Geometry check sheet. Reference: the model listing, model coordinates, mm. A direction names the side the tool comes from. Coordinates: 2 decimals unless noted, no trailing zeros. Loops run counter-clockwise (first coordinate to the right, second up) from the corner with the lowest first, then second, coordinate; pieces in that order, holes last. Notation, with made-up numbers: (9, 23) - (44, 23) arc R19 cw to (44, 39) - close; hole circle Ø1 at (-4.75, 42). An arc over 180 degrees is marked (long way). One line per item, written item: value.
Autodesk Inventor part; units mm, degrees
ref_plane "YZ Plane" through (0, 0, 0) normal (1, 0, 0) x (0, 1, 0)
ref_plane "XZ Plane" through (0, 0, 0) normal (0, 1, 0) x (-1, 0, 0)
ref_plane "XY Plane" through (0, 0, 0) normal (0, 0, 1) x (1, 0, 0)
sketch "Sketch1" plane through (0, 0, 0) normal (0, 1, 0) x (-1, 0, 0)
  line L0 (0, 0) -> (15, 0)
  line L1 (15, 0) -> (15, -32)
  line L2 (15, -32) -> (0, -32)
  line L3 (0, -32) -> (0, 0)
  line L4 (3, 0) -> (12, 0)
  line L5 (12, 0) -> (12, 8)
  line L6 (12, 8) -> (3, 8)
  line L7 (3, 8) -> (3, 0)
  line L8 (-5, -32) -> (-5, 5)
  line L9 (-5, 5) -> (-2, 5)
  line L10 (-2, 5) -> (-2, 13)
  line L11 (-2, 13) -> (17, 13)
  line L12 (17, 13) -> (17, 5)
  line L13 (17, 5) -> (20, 5)
  line L14 (20, 5) -> (20, -37)
  line L15 (20, -37) -> (-5, -37)
  line L16 (-5, -37) -> (-5, -32)
  line L17 (-5, -8.634) -> (-25, -8.634)
  line L18 (-25, -8.634) -> (-25, -18.634)
  line L19 (-25, -18.634) -> (-5, -18.634)
  line L20 (-5, -18.634) -> (-5, -8.634)
  line L21 (20, -18.634) -> (40, -18.634)
  line L22 (40, -18.634) -> (40, -8.634)
  line L23 (40, -8.634) -> (20, -8.634)
  line L24 (20, -8.634) -> (20, -18.634)
  dimension "d0" = 15
  dimension "d1" = 32
  dimension "d2" = 9
  dimension "d3" = 3
  dimension "d4" = 3
  dimension "d5" = 8
  dimension "d6" = 5
  dimension "d7" = 5
  dimension "d8" = 5
  dimension "d9" = 5
  dimension "d10" = 5
  dimension "d11" = 5
  dimension "d12" = 5
  dimension "d13" = 5
  dimension "d71" = 20
  dimension "d72" = 10
  dimension "d73" = 20
  dimension "d74" = 10
extrude "Extrusion1" add sketch "Sketch1" along normal blind 10
sketch "Sketch3" plane through (5, 0, -37) normal (0, 0, -1) x (-1, 0, 0)
  line L0 (0.5, 10) -> (24.5, 10)
  line L1 (24.5, 10) -> (24.5, 1)
  line L2 (24.5, 1) -> (0.5, 1)
  line L3 (0.5, 1) -> (0.5, 10)
  line L4 (25, 0) -> (25, 10)
  line L5 (0, 0) -> (0, 10)
  line L6 (0, 0) -> (25, 0)
  line L7 (0, 10) -> (25, 10)
  point P0 (5, 0)
  point P1 (24.5, 5.5)
  dimension "d24" = 0.5
  dimension "d25" = 0.5
  dimension "d26" = 1
  dimension "d27" = 0
extrude "Extrusion3" cut sketch "Sketch3" against normal blind 10 contours L0 L1 L2 L3
sketch "Sketch4" plane through (-17, 0, 13) normal (0, 0, 1) x (1, 0, 0)
  line L0 (5, 10) -> (14, 10)
  line L1 (14, 10) -> (14, 2)
  line L2 (14, 2) -> (5, 2)
  line L3 (5, 2) -> (5, 10)
  line L4 (0, 0) -> (19, 0)
  line L5 (0, 10) -> (19, 10)
  line L6 (19, 0) -> (19, 10)
  line L7 (0, 0) -> (0, 10)
  point P0 (17, 0)
  point P1 (9.5, 0)
  dimension "d30" = 2
  dimension "d31" = 0
  dimension "d32" = 5
  dimension "d33" = 5
extrude "Extrusion4" cut sketch "Sketch4" against normal blind 10 contours L0 L1 L2 L3
sketch "Sketch5" plane through (0, 0, 0) normal (0, -1, 0) x (1, 0, 0)
  line L0 (-17, 5) -> (-17, 13)
  line L1 (2, 13) -> (2, 5)
  line L2 (-17, 13) -> (2, 13)
  line L3 (2, 13) -> (2, 5)
  line L4 (5, 5) -> (5, -37)
  line L5 (2, 5) -> (5, 5)
  line L6 (5, 5) -> (5, -37)
  line L7 (-20, -37) -> (-20, 5)
  line L8 (5, -37) -> (-20, -37)
  line L9 (-20, -37) -> (-20, 5)
  line L10 (-20, 5) -> (-17, 5)
  point P0 (0, 0)
extrude "Extrusion5" add sketch "Sketch5" along normal blind 5
sketch "Sketch6" plane through (0, 10, 0) normal (0, 1, 0) x (1, 0, 0)
  circle A0 centre (-18.5, 2.5) radius 1
  line L0 (-20, -5) -> (-17, -5)
  line L1 (-20, 37) -> (-20, -5)
  circle A1 centre (3.5, 2.5) radius 1
  line L2 (2, -5) -> (5, -5)
  line L3 (2, -13) -> (2, -5)
  point P0 (0, 0)
  dimension "d59" = 2
  dimension "d60" = 7.5
  dimension "d61" = 1.5
  dimension "d62" = 2
  dimension "d63" = 7.5
  dimension "d64" = 1.5
extrude "Extrusion6" cut sketch "Sketch6" against normal blind 5
thread "Thread1"
thread "Thread2"
sketch "Sketch7" plane through (25, 0, -18.634) normal (0, 0, -1) x (-1, 0, 0)
  point P0 (25, 0)
sketch "Sketch8" plane through (25, 0, -18.634) normal (0, 0, -1) x (-1, 0, 0)
  circle A0 centre (10, 5) radius 2
  circle A1 centre (55, 5) radius 2
  line L0 (65, 0) -> (65, 10)
  line L1 (0, 0) -> (0, 10)
  line L2 (0, 10) -> (20, 10)
  line L3 (45, 10) -> (65, 10)
  point P0 (25, 0)
  point P1 (65, 5)
  dimension "d76" = 4
  dimension "d77" = 4
  dimension "d78" = 10
  dimension "d79" = 10
  dimension "d80" = 5
  dimension "d81" = 5
extrude "Extrusion7" cut sketch "Sketch8" against normal blind 10
thread "Thread3"
thread "Thread4"
properties part number "Base"
(1) Release check for a two-part mould opening along Z. For faces 1 (the face through (-8, 1, 8)), 2 (the face through (-17, 6, -27)), 3 (the face through (15, 0, -14)) record: pulls with the +Z half, pulls with the -Z half, needs draft (parallel to the pull), parting line crosses it, or undercut.
Reply:
face 1: undercut
face 2: pulls with the -Z half
face 3: needs draft
(2) Cross-section at D-D on x = 3.5. Record the cut outline in (y, z).
Reply:
outline: (-5, -37) - (1, -37) - (1, -27) - (10, -27) - (10, -3.5) - (5, -3.5) - (5, -1.5) - (10, -1.5) - (10, 5) - (-5, 5) - close
(3) Cross-section at C-C on z = -13. Record the cut outline in (x, y), and give its area (3 significant figures).
Reply:
outline: (-40, 0) - (-20, 0) - (-20, -5) - (5, -5) - (5, 0) - (25, 0) - (25, 10) - (0, 10) - (0, 0) - (-15, 0) - (-15, 10) - (-40, 10) - close; hole circle Ø4 at (-30, 5); hole circle Ø4 at (15, 5)
area: 600 mm2
(4) Cross-section at A-A on y = 9. State how many separate pieces and enclosed holes the cut face has, and give its area (3 significant figures).
Reply:
separate pieces: 2
enclosed holes: 2
area: 834 mm2
(5) Go/stop test with flat-tipped pins: pin 1 Ø3.5 at (x, y) = (15, 5) entering from +Z; pin 2 Ø1 at (y, z) = (1, -5) entering from +X; pin 3 Ø1.3 at (x, y) = (2.5, 7) entering from -Z; pin 4 Ø4 at (x, y) = (-31.5, -1) entering from +Z. Record where each tip stops, or that it passes through.
Reply:
pin 1: through
pin 2: x = 5
pin 3: z = -27
pin 4: z = -8.63
(6) Cross-section at B-B on x = -30. Record the cut outline in (y, z).
Reply:
outline: (0, -18.63) - (3, -18.63) - (3, -8.63) - (0, -8.63) - close; (7, -18.63) - (10, -18.63) - (10, -8.63) - (7, -8.63) - close
(7) Access from +Z, -Z, +X, -X, +Y, -Y to the whole of each face (thin tool, end or side, straight path). Record for faces 4 (the face through (-27.6, 4.9, -18.634)), 5 (the face through (12.6, 4.9, -8.634)), 6 (the face through (17.4, 4.9, -18.634)), 7 (the face through (-30, 0, -14)).
Reply:
face 4: -Z, -X, +Y, -Y
face 5: +Z, +X, +Y, -Y
face 6: -Z, +X, +Y, -Y
face 7: +Z, -Z, -X, -Y
(8) Material ranges on probe 1 along X at (y, z) = (7.5, -2.5); probe 2 along X at (y, z) = (5.25, -17.5); probe 3 along Z at (x, y) = (-18.5, 7.05), recorded low to high. Write a range as from..to.
Reply:
probe 1: -20..-19.5, -17.5..-15, 0..2.5, 4.5..5
probe 2: -40..-31.98, -28.02..-15, 0..13.02, 16.98..25
probe 3: -27..-3.5, -1.5..5
